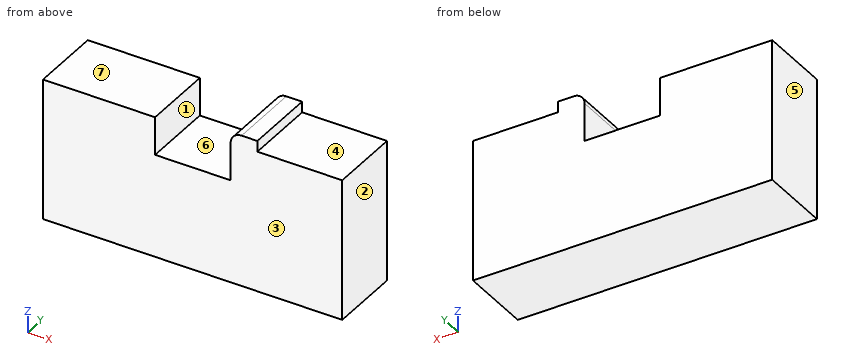
from build123d import *

# Parameters (mm, degrees)
F0_W     = 69.85
F0_H     = 33.02
F1_DEPTH = 16.891
F2_W     = 17.653
F2_H     = 8.89
F3_DEPTH = 25.4
F4_W     = 6.223
F4_H     = 16.891
F5_DEPTH = 2.54
F6_R     = 2.54


with BuildPart() as f1:
    # F0 (on Front) → F1 (new body)
    with BuildSketch(Plane.XZ):
        with Locations((34.925, 16.51)):
            Rectangle(F0_W, F0_H)
    extrude(amount=F1_DEPTH)

    # F2 (on face) → F3 (cut)
    with BuildSketch(Plane.XZ.offset(16.891)):
        with Locations((34.9885, 28.575)):
            Rectangle(F2_W, F2_H)
    extrude(amount=-F3_DEPTH, mode=Mode.SUBTRACT)

    # F4 (on face) → F5 (join)
    with BuildSketch(Plane.XY.offset(33.02)):
        with Locations((46.9265, -8.4455)):
            Rectangle(F4_W, F4_H)
    extrude(amount=F5_DEPTH)

    # F6
    f6_edges = [f1.edges().sort_by_distance(p)[0] for p in [
        (43.815, -8.4455, 35.56),
    ]]
    fillet(f6_edges, radius=F6_R)


solid = f1.part
Source: CAD feature listing. Evaluate the final solid. Frame: model axes, mm. Face numbers are marked on the shaded views. A direction names the side the tool comes from. Round coordinates to 2 decimals unless told otherwise and drop trailing zeros. Loops run counter-clockwise (first coordinate to the right, second up) from the corner with the lowest first, then second, coordinate; pieces in that order, holes last.
Q1. Section A-A, the plane z = 28. Return loops of the section in (x, y) (3 decimals).
Q2. Ray query, line 1 (X direction, y = -5.5, z = 29) (3 decimals); line 2 (Z direction, x = 29.5, y = -5.5); line 3 (Z direction, x = 65, y = -8.25). Return the intervals inside material, ascending.
Q3. Mould query, pull axis X, two halves, no side actions, for the marked faces 1, 2 and 3. Classes: pulls with the +X half, pulls with the -X half, needs draft (parallel to the pull), parting line crosses it, or undercut.
Q4. Access query for the marked faces 4, 5, 6 and 7. Directions: +Z, -Z, +X, -X, +Y, -Y. A direction counts if a zero-diameter tool reaches every point of the face in a straight line with its end or side. Return the directions, or none.
Q5. First-contact query: P1, Ø3, axis at x = 41.5, y = -9, coming from the +Z side; P2, Ø8.5, axis at x = 63, y = -5.5, coming from the +Z side. Flat tips, straight axial feed; report the tip coordinate or a pass-through.
Q6. Section B-B, the plane y = -6.25. Return loops of the section in (x, z) (3 decimals), plus the area to 3 significant figures.
Q7. Section C-C, the plane x = 14.5. Return loops of the section in (y, z), plus the area to 3 significant figures.
Solutions:
1. outline: (0, -16.891) - (26.162, -16.891) - (26.162, 0) - (0, 0) - close; (43.815, -16.891) - (69.85, -16.891) - (69.85, 0) - (43.815, 0) - close
2. line 1: x = 0 to 26.162, 43.815 to 69.85
2. line 2: z = 0 to 24.13
2. line 3: z = 0 to 33.02
3. face 1: undercut
3. face 2: pulls with the +X half
3. face 3: needs draft
4. face 4: +Z, +X, +Y, -Y
4. face 5: +Z, -Z, -X, +Y, -Y
4. face 6: +Z, +Y, -Y
4. face 7: +Z, -X, +Y, -Y
5. P1: stops at z = 24.13
5. P2: stops at z = 33.02
6. outline: (0, 0) - (69.85, 0) - (69.85, 33.02) - (50.038, 33.02) - (50.038, 35.56) - (46.355, 35.56) arc R2.54 ccw to (43.815, 33.02) - (43.815, 24.13) - (26.162, 24.13) - (26.162, 33.02) - (0, 33.02) - close
6. area: 2,160 mm2
7. outline: (-16.89, 0) - (0, 0) - (0, 33.02) - (-16.89, 33.02) - close
7. area: 558 mm2
